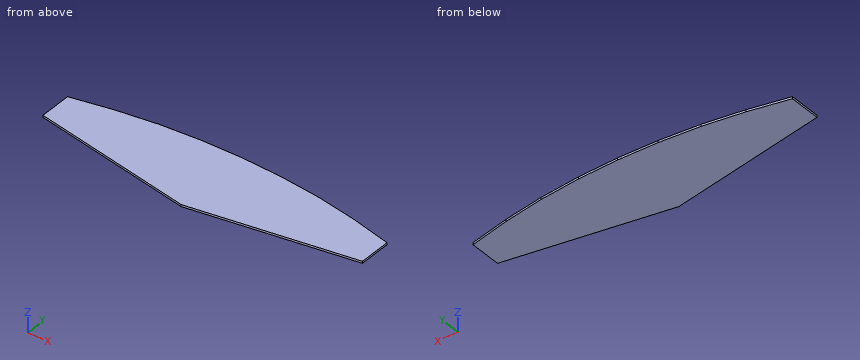
from build123d import *

# Parameters (mm, degrees)
F1_DEPTH = 5


with BuildPart() as f1:
    # F0 (on Top) → F1 (new body)
    with BuildSketch(Plane.XY):
        Polygon((404, 70), (404, 150), (303, 172), (303, 52.5), align=None)
        Polygon((303, 52.5), (303, 172), (202, 188), (202, 35), align=None)
        Polygon((202, 35), (202, 188), (101, 197), (101, 17.5), align=None)
        Polygon((101, 17.5), (101, 197), (0, 200), (0, 0), align=None)
        Polygon((0, 0), (0, 200), (-101, 197), (-101, 17.5), align=None)
        Polygon((-101, 17.5), (-101, 197), (-202, 188), (-202, 35), align=None)
        Polygon((-202, 35), (-202, 188), (-303, 172), (-303, 52.5), align=None)
        Polygon((-303, 52.5), (-303, 172), (-404, 150), (-404, 70), align=None)
    extrude(amount=F1_DEPTH)


solid = f1.part
Build history of the part. All positions in model axes, mm. Give positions to 0.01 mm unless a question says otherwise; leave off trailing zeros. Write each loop counter-clockwise with the first axis right and the second up, starting at its lowest first coordinate (ties: lowest second). Pieces come first, ordered by that corner, then holes. Notation, with made-up numbers: (68, -24) - (81, -24) arc R32 ccw to (81, 10) - close; hole circle Ø1 at (25, 17.25). An arc over 180 degrees is marked (long way). Use one line per item in the form item = value. Start each with the question number.
1. Band-saw the part on B-B on y = 63. Write the cut outline in (x, z).
2. Probe line 1 (Y direction, x = -229.5, z = 3.2); line 2 (Y direction, x = -199.5, z = 2.85). List the from-to ranges inside material, lowest first. Write a range as [from, to].
3. Band-saw the part on A-A on z = 1.55. Write the cut outline in (x, y), plus the area to 3 significant figures.
4. Band-saw the part on C-C on x = -192. Write the cut outline in (y, z).
Conclusion:
q1.outline = (-363.6, 0) - (363.6, 0) - (363.6, 5) - (-363.6, 5) - close
q2.line_1 = [39.76, 183.64]
q2.line_2 = [34.57, 188.22]
q3.outline = (-404, 70) - (0, 0) - (404, 70) - (404, 150) - (303, 172) - (202, 188) - (101, 197) - (0, 200) - (-101, 197) - (-202, 188) - (-303, 172) - (-404, 150) - close
q3.area = 120,000 mm²
q4.outline = (33.27, 0) - (188.89, 0) - (188.89, 5) - (33.27, 5) - close
